Model file for the job. Use its own axes, mm. Face numbers are marked on the shaded views. A direction names the side the tool comes from. Coordinates: 2 decimals unless noted, no trailing zeros. Write each loop counter-clockwise with the first axis right and the second up, starting at its lowest first coordinate (ties: lowest second). Pieces come first, ordered by that corner, then holes. Notation, with made-up numbers: M -16,22 L 17,22 A22 cw 17,51 Z; hole C 77.5,89 d6. An arc over 180 degrees is marked long. Put each result on its own line as item: value. Start each with the question number.
Q1. Which spindle directions (+Z, -Z, +X, -X, +Y, -Y) get a long thin tool onto all of the face, cutting with end or side? Do the marked faces 1, 2 and 3. Say none if no direction does.
Q2. Cut at C-C (z = 7.5). Write the cut outline in (x, y), then the cut area to 3 significant figures.
Q3. Cut at D-D (x = 7). Write the cut outline in (y, z).
Q4. Cut at A-A (x = 0). Write the cut outline in (y, z), then the cut area to 3 significant figures.
Q5. Drop flat-ended pins along their axis: pin 1 (3.5 mm diameter, centred on x = -8, z = 7.5, fed in from +Y); pin 2 (4.5 mm diameter, centred on x = 7.5, z = 7, fed in from -Y); pin 3 (5 mm diameter, centred on x = 5, y = 30, fed in from +Z); pin 4 (2.5 mm diameter, centred on x = -7, y = 41.3, fed in from +Z). Give the stop position or say it passes through.
Q6. Cut at B-B (y = 39). Write the cut outline in (x, z), then the cut area to 3 significant figures.
Q7. Pull direction X, two halves, no side cores. Call the marked faces 4, 5 and 6: pulls with the +X half, pulls with the -X half, needs draft (parallel to the pull), parting line crosses it, or undercut.
Q8. Drill centre lines: line 1 along Y through (x, z) = (0, -10); line 2 along X through (y, z) = (4.75, 7.5); line 3 along Y through (x, z) = (-6, 0.5). Where is each one in solid material? Low to high.
```python
from build123d import *

# Parameters (mm, degrees)
CROQUIS1_W              = 32
CROQUIS1_H              = 32
SALIENTE_EXTRUIR1_DEPTH = 42
CORTAR_EXTRUIR1_DEPTH   = 42
CROQUIS3_W              = 8
CROQUIS3_H              = 0.624082803
CORTAR_EXTRUIR2_DEPTH   = 42
CORTAR_EXTRUIR3_DEPTH   = 55.698871322
CROQUIS7_R              = 11.922640385
SALIENTE_EXTRUIR3_DEPTH = 8
CROQUIS8_R              = 3
CROQUIS8_R_2            = 1.5
CORTAR_EXTRUIR5_DEPTH   = 61.603104214
CROQUIS9_R              = 2.05
CORTAR_EXTRUIR6_DEPTH   = 6


with BuildPart() as part:
    # Croquis1 → Saliente-Extruir1 (new body)
    with BuildSketch(Plane(origin=(0, 0, 0), x_dir=(1, 0, 0), z_dir=(0, 1, 0))):
        Rectangle(CROQUIS1_W, CROQUIS1_H)
    extrude(amount=SALIENTE_EXTRUIR1_DEPTH)

    # Croquis2 → Cortar-Extruir1 (cut)
    with BuildSketch(Plane(origin=(16, 0, 0), x_dir=(0, 0, -1), z_dir=(1, 0, 0))):
        Polygon((-16, 12.058), (3, 12.058), (8, 17.081917197), (8, 42), (-16, 42), align=None)
    extrude(amount=-CORTAR_EXTRUIR1_DEPTH, mode=Mode.SUBTRACT)

    # Croquis3 → Cortar-Extruir2 (cut)
    with BuildSketch(Plane(origin=(16, 0, 0), x_dir=(0, 0, -1), z_dir=(1, 0, 0))):
        with Locations((12, 41.687958599)):
            Rectangle(CROQUIS3_W, CROQUIS3_H)
    extrude(amount=-CORTAR_EXTRUIR2_DEPTH, mode=Mode.SUBTRACT)

    # Croquis6 → Cortar-Extruir3 (cut, through all)
    with BuildSketch(Plane.XY.offset(16)):
        Polygon((-16, 0), (-11.922640385, 41.375917197), (-16, 41.375917197), align=None)
        Polygon((16, 0), (11.922640385, 41.375917197), (16, 41.375917197), align=None)
    extrude(amount=-CORTAR_EXTRUIR3_DEPTH, mode=Mode.SUBTRACT)

    # Croquis7 → Saliente-Extruir3 (add)
    with BuildSketch(Plane(origin=(0, 0, -16), x_dir=(-1, 0, 0), z_dir=(0, 0, -1))):
        with Locations((0, 41.375917197)):
            Circle(CROQUIS7_R)
    extrude(amount=-SALIENTE_EXTRUIR3_DEPTH)

    # Croquis8 → Cortar-Extruir5 (cut, through all)
    with BuildSketch(Plane.XY.offset(-8)):
        with Locations((0, 41.298557582)):
            Circle(CROQUIS8_R)
        with Locations((1.182e-06, 48.298557582)):
            Circle(CROQUIS8_R_2)
        with Locations((7, 41.2985564)):
            Circle(CROQUIS8_R_2)
        with Locations((-1.182e-06, 34.298557582)):
            Circle(CROQUIS8_R_2)
        with Locations((-7, 41.298558764)):
            Circle(CROQUIS8_R_2)
    extrude(amount=-CORTAR_EXTRUIR5_DEPTH, mode=Mode.SUBTRACT)

    # Croquis9 → Cortar-Extruir6 (cut)
    with BuildSketch(Plane.XZ):
        with Locations(Location((-8, 7.5, 0), (0, 0, 270))):
            Circle(CROQUIS9_R)
        with Locations(Location((8, 7.5, 0), (0, 0, 270))):
            Circle(CROQUIS9_R)
    extrude(amount=-CORTAR_EXTRUIR6_DEPTH, mode=Mode.SUBTRACT)


solid = part.part
```
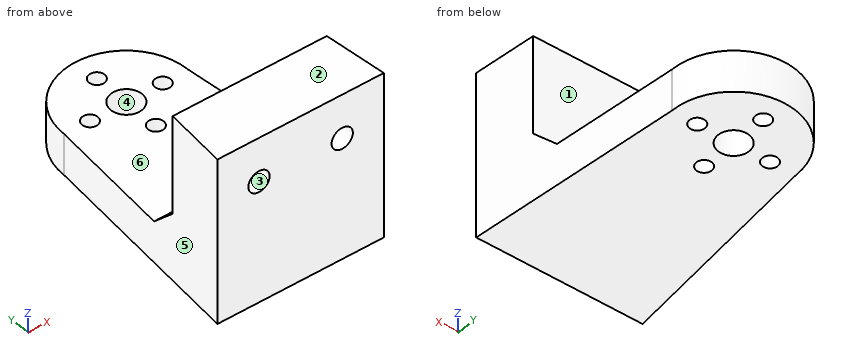
Computed values:
1. face 1: +Z, +X, -X, +Y
1. face 2: +Z, +X, -X, +Y, -Y
1. face 3: -Y
2. outline: M -16,0 L -10.05,0 L -10.05,6 L -5.95,6 L -5.95,0 L 5.95,0 L 5.95,6 L 10.05,6 L 10.05,0 L 16,0 L 14.81,12.06 L -14.81,12.06 Z
2. area: 322 mm2
3. outline: M 0,-16 L 39.8,-16 L 39.8,-8 L 17.08,-8 L 12.06,-3 L 12.06,16 L 0,16 L 0,9.29 L 6,9.29 L 6,5.71 L 0,5.71 Z; M 42.8,-16 L 51.03,-16 L 51.03,-8 L 42.8,-8 Z
4. outline: M 0,-16 L 32.8,-16 L 32.8,-8 L 17.08,-8 L 12.06,-3 L 12.06,16 L 0,16 Z; M 35.8,-16 L 38.3,-16 L 38.3,-8 L 35.8,-8 Z; M 44.3,-16 L 46.8,-16 L 46.8,-8 L 44.3,-8 Z; M 49.8,-16 L 53.3,-16 L 53.3,-8 L 49.8,-8 Z
4. area: 632 mm2
5. pin 1: y = 12.06
5. pin 2: y = 0
5. pin 3: z = -8
5. pin 4: through
6. outline: M -12.16,-16 L -1.93,-16 L -1.93,-8 L -12.16,-8 Z; M 1.93,-16 L 12.16,-16 L 12.16,-8 L 1.93,-8 Z
6. area: 164 mm2
7. face 4: undercut
7. face 5: pulls with the -X half
7. face 6: needs draft
8. line 1: 0 to 32.8, 35.8 to 38.3, 44.3 to 46.8, 49.8 to 53.3
8. line 2: -15.53 to -10.05, -5.95 to 5.95, 10.05 to 15.53
8. line 3: 0 to 12.06
